Autodesk Inventor part; units mm, degrees
ref_plane "YZ Plane" through (0, 0, 0) normal (1, 0, 0) x (0, 1, 0)
ref_plane "XZ Plane" through (0, 0, 0) normal (0, 1, 0) x (-1, 0, 0)
ref_plane "XY Plane" through (0, 0, 0) normal (0, 0, 1) x (1, 0, 0)
sketch "Sketch1" plane through (0, 0, 0) normal (1, 0, 0) x (0, 1, 0)
  line L0 (0, 0) -> (0, -10)
  line L1 (0, -10) -> (10, -10)
  line L2 (10, -10) -> (10, -8.5)
  line L3 (0, 0) -> (10, 0)
  line L4 (10, 0) -> (10, -1.5)
  line L5 (0, -5) -> (1.5, -5) construction
  line L6 (10, -1.5) -> (1.5, -1.5)
  line L7 (1.5, -1.5) -> (1.5, -8.5)
  line L8 (1.5, -8.5) -> (10, -8.5)
  dimension "d0" = 10
  dimension "d1" = 10
  dimension "d2" = 1.5
  dimension "d3" = 10
  dimension "d4" = 1.5
  dimension "d5" = 1.5
extrude "Extrusion1" add sketch "Sketch1" along normal blind 660.4
properties part number "26in mini C-Channel (rail)" material "Aluminum 6061"
Build history of the part. All positions in model axes, mm. Give positions to 0.01 mm unless a question says otherwise; leave off trailing zeros. Order: outer loops, then holes, each group sorted by start corner. A loop starts at its lowest first (then second) coordinate and runs counter-clockwise, first axis right, second up. Notation, with made-up numbers: M 75.5,30 L 122.5,30 A4 cw 122.5,35 Z; hole C 20.25,68.5 d8. An arc over 180 degrees is marked long. Write item = value, one per line. Start each with the question number.
(1) Slice it at B-B on x = 200.5. Write the cut outline in (y, z).
(2) Slice it at C-C on z = -5.5. Write the cut outline in (x, y).
(3) Pin check, flat tip, straight feed: pin 1 Ø3.5 at (x, z) = (318.5, -3.5) entering from +Y. Stop position of the tip, or through.
(4) Slice it at A-A on y = 4.25. Write the cut outline in (x, z), plus the area to 3 significant figures.
(5) Probe L1, parallel to Z at x = 54, y = 8.25; L2, parallel to Y at x = 248, z = -5.25. List the from-to ranges inside material, lowest first. Write a range as [from, to].
Responses:
q1.outline = M 0,-10 L 10,-10 L 10,-8.5 L 1.5,-8.5 L 1.5,-1.5 L 10,-1.5 L 10,0 L 0,0 Z
q2.outline = M 0,0 L 660.4,0 L 660.4,1.5 L 0,1.5 Z
q3.pin_1 = 1.5
q4.outline = M 0,-10 L 660.4,-10 L 660.4,-8.5 L 0,-8.5 Z; M 0,-1.5 L 660.4,-1.5 L 660.4,0 L 0,0 Z
q4.area = 1,980 mm2
q5.L1 = [-10, -8.5], [-1.5, 0]
q5.L2 = [0, 1.5]
